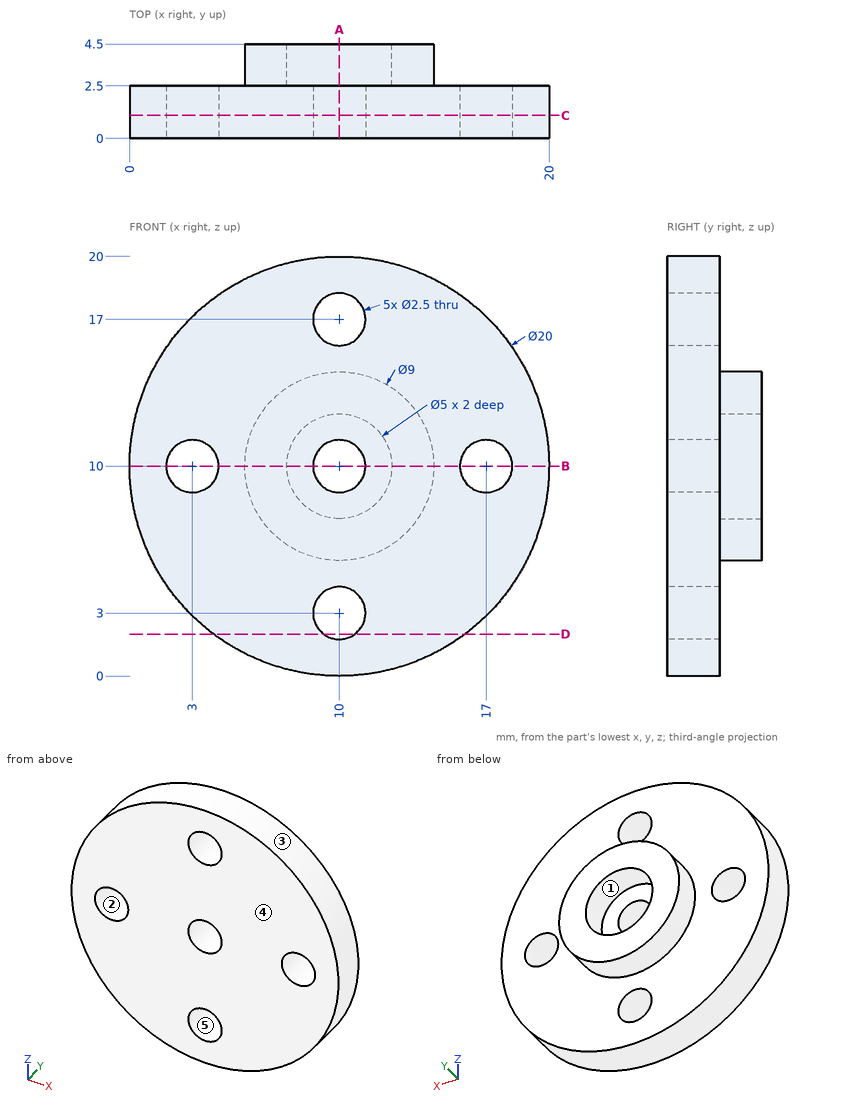
Here's the drawing with two shaded views (mm, measured from the low corner). I have some questions. A direction names the side the tool comes from. Round coordinates to 2 decimals unless told otherwise and drop trailing zeros. Loops run counter-clockwise (first coordinate to the right, second up) from the corner with the lowest first, then second, coordinate; pieces in that order, holes last. Notation, with made-up numbers: M -26.75,58.25 L -14.75,58.25 A28 cw -14.75,84.25 Z; hole C 19,2 d9. An arc over 180 degrees is marked long. Answer as a JSON object with one key per item and string values. Group by question number.
Q1. Imagine slicing it at D-D, the plane z = 2. Please give me the cut outline in (x, y).
Q2. Imagine slicing it at B-B, the plane z = 10. Please give me the cut outline in (x, y), then the cut area to 4 significant figures.
Q3. On a 3-axis mill with a long thin cutter (end or side, diameter ignored), from which of +Z, -Z, +X, -X, +Y, -Y can I reach the whole of each face in a straight line? I mean the marked faces 1 and 2. Say none if no direction works.
Q4. Imagine slicing it at A-A, the plane x = 10. Please give me the cut outline in (y, z), then the cut area to 4 significant figures.
Q5. Imagine slicing it at C-C, the plane y = 1.1. Please give me the cut outline in (x, z), then the cut area to 3 significant figures.
Q6. Will these pins go through, and if not, where does the flat tip stop? pin 1 (2 mm diameter, centred on x = 17, z = 10, fed in from -Y) (3 decimals); pin 2 (1.5 mm diameter, centred on x = 13.5, y = 3.5, fed in from +Z).
Q7. Please list where these lines run through material, in increasing order: L1, parallel to X at y = 0.55, z = 10; L2, parallel to X at y = 3.45, z = 10.
Q8. We'd pull the mould along X, two halves only. Please class the marked faces 3, 4 and 5: +X half, -X half, draft (parallel to the pull), parting line (faces both ways), or undercut.
Findings:
{
 "1": {"outline": "M 4,0 L 9.25,0 L 9.25,2.5 L 4,2.5 Z; M 10.75,0 L 16,0 L 16,2.5 L 10.75,2.5 Z"},
 "2": {"outline": "M 0,0 L 1.75,0 L 1.75,2.5 L 0,2.5 Z; M 4.25,0 L 8.75,0 L 8.75,2.5 L 7.5,2.5 L 7.5,4.5 L 5.5,4.5 L 5.5,2.5 L 4.25,2.5 Z; M 11.25,0 L 15.75,0 L 15.75,2.5 L 14.5,2.5 L 14.5,4.5 L 12.5,4.5 L 12.5,2.5 L 11.25,2.5 Z; M 18.25,0 L 20,0 L 20,2.5 L 18.25,2.5 Z", "area": "39.25 mm2"},
 "3": {"face 1": "+Y", "face 2": "+Y, -Y"},
 "4": {"outline": "M 0,0 L 2.5,0 L 2.5,1.75 L 0,1.75 Z; M 0,4.25 L 2.5,4.25 L 2.5,5.5 L 4.5,5.5 L 4.5,7.5 L 2.5,7.5 L 2.5,8.75 L 0,8.75 Z; M 0,11.25 L 2.5,11.25 L 2.5,12.5 L 4.5,12.5 L 4.5,14.5 L 2.5,14.5 L 2.5,15.75 L 0,15.75 Z; M 0,18.25 L 2.5,18.25 L 2.5,20 L 0,20 Z", "area": "39.25 mm2"},
 "5": {"outline": "C 10,10 d20; hole C 3,10 d2.5; hole C 10,3 d2.5; hole C 10,10 d2.5; hole C 10,17 d2.5; hole C 17,10 d2.5", "area": "290 mm2"},
 "6": {"pin 1": "passes through", "pin 2": "stops at z = 13.56"},
 "7": {"L1": "x = 0 to 1.75, 4.25 to 8.75, 11.25 to 15.75, 18.25 to 20", "L2": "x = 5.5 to 7.5, 12.5 to 14.5"},
 "8": {"face 3": "parting line", "face 4": "draft", "face 5": "undercut"}
}
